```python
from build123d import *

# Parameters (mm, degrees)
F0_W      = 70
F0_H      = 100
F1_DEPTH  = 45
F2_W      = 60
F2_H      = 90
F3_DEPTH  = 40
F4_R      = 2.65
F5_DEPTH  = 5
F6_DEPTH  = 25
F7_DEPTH  = 25
F8_DEPTH  = 25
F9_W      = 5
F9_H      = 100
F10_DEPTH = 25
F11_W     = 5
F11_H     = 100
F12_DEPTH = 25
F14_DEPTH = 25
F15_DEPTH = 25
F17_DEPTH = 25
F18_W     = 67
F18_H     = 97
F18_W_2   = 63
F18_H_2   = 93
F19_DEPTH = 2
F13_W     = 5
F13_H     = 30
F20_DEPTH = 25
F16_W     = 5
F16_H     = 30
F21_DEPTH = 25
F22_R     = 5
F23_DEPTH = 25
F25_DEPTH = 100


with BuildPart() as f1:
    # F0 (on Front) → F1 (new body)
    with BuildSketch(Plane.XZ):
        with Locations((12.707982, -8.253274)):
            Rectangle(F0_W, F0_H)
    extrude(amount=F1_DEPTH)

    # F2 (on face) → F3 (cut)
    with BuildSketch(Plane.XZ.offset(45)):
        with Locations((12.707982, -8.253274)):
            Rectangle(F2_W, F2_H)
    extrude(amount=-F3_DEPTH, mode=Mode.SUBTRACT)

    # F4 (on face) → F5 (cut)
    with BuildSketch(Plane.XZ.offset(5)):
        with Locations((-9.792018, 29.246726)):
            Circle(F4_R)
    extrude(amount=-F5_DEPTH, mode=Mode.SUBTRACT)

    # F4 (on face) → F6 (cut)
    with BuildSketch(Plane.XZ.offset(5)):
        with Locations((35.207982, 29.246726)):
            Circle(F4_R)
    extrude(amount=-F6_DEPTH, mode=Mode.SUBTRACT)

    # F4 (on face) → F7 (cut)
    with BuildSketch(Plane.XZ.offset(5)):
        with Locations((35.207982, -45.753274)):
            Circle(F4_R)
    extrude(amount=-F7_DEPTH, mode=Mode.SUBTRACT)

    # F4 (on face) → F8 (cut)
    with BuildSketch(Plane.XZ.offset(5)):
        with Locations((-9.792018, -45.753274)):
            Circle(F4_R)
    extrude(amount=-F8_DEPTH, mode=Mode.SUBTRACT)

    # F9 (on face) → F10 (join)
    with BuildSketch(Plane(origin=(-22.292018, 0, 0), x_dir=(0, -1, 0), z_dir=(-1, 0, 0))):
        with Locations((2.5, -8.253274)):
            Rectangle(F9_W, F9_H)
    extrude(amount=F10_DEPTH)

    # F11 (on face) → F12 (join)
    with BuildSketch(Plane.YZ.offset(47.707982)):
        with Locations((-2.5, -8.253274)):
            Rectangle(F11_W, F11_H)
    extrude(amount=F12_DEPTH)

    # F13 (on face) → F14 (cut)
    with BuildSketch(Plane.XZ.offset(5)):
        with BuildLine():
            ThreePointArc((-47.292018, 16.746726), (-39.969687, 34.424395), (-22.292018, 41.746726))
            Line((-22.292018, 41.746726), (-47.292018, 41.746726))
            Line((-47.292018, 41.746726), (-47.292018, 16.746726))
        make_face()
    extrude(amount=-F14_DEPTH, mode=Mode.SUBTRACT)

    # F13 (on face) → F15 (cut)
    with BuildSketch(Plane.XZ.offset(5)):
        with BuildLine():
            Line((-47.292018, -58.253274), (-22.292018, -58.253274))
            ThreePointArc((-22.292018, -58.253274), (-39.969687, -50.930944), (-47.292018, -33.253274))
            Line((-47.292018, -33.253274), (-47.292018, -58.253274))
        make_face()
    extrude(amount=-F15_DEPTH, mode=Mode.SUBTRACT)

    # F16 (on face) → F17 (cut)
    with BuildSketch(Plane.XZ.offset(5)):
        with BuildLine():
            Line((72.707982, 41.746726), (47.707982, 41.746726))
            ThreePointArc((47.707982, 41.746726), (65.385652, 34.424395), (72.707982, 16.746726))
            Line((72.707982, 16.746726), (72.707982, 41.746726))
        make_face()
        with BuildLine():
            ThreePointArc((72.707982, -33.253274), (65.385652, -50.930944), (47.707982, -58.253274))
            Line((47.707982, -58.253274), (72.707982, -58.253274))
            Line((72.707982, -58.253274), (72.707982, -33.253274))
        make_face()
    extrude(amount=-F17_DEPTH, mode=Mode.SUBTRACT)

    # F18 (on face) → F19 (cut)
    with BuildSketch(Plane.XZ.offset(45)):
        with Locations((12.707982, -8.253274)):
            Rectangle(F18_W, F18_H)
        with Locations((12.707982, -8.253274)):
            Rectangle(F18_W_2, F18_H_2, mode=Mode.SUBTRACT)
    extrude(amount=-F19_DEPTH, mode=Mode.SUBTRACT)

    # F13 (on face) → F20 (cut)
    with BuildSketch(Plane.XZ.offset(5)):
        Polygon((-37.292018, 6.746726), (-42.292018, 6.746726), (-42.292018, -23.253274), (-37.288308, -23.253274), align=None)
        with Locations((-29.792018, -8.253274)):
            Rectangle(F13_W, F13_H)
    extrude(amount=-F20_DEPTH, mode=Mode.SUBTRACT)

    # F16 (on face) → F21 (cut)
    with BuildSketch(Plane.XZ.offset(5)):
        with Locations((55.207982, -8.253274)):
            Rectangle(F16_W, F16_H)
        with Locations((65.207982, -8.253274)):
            Rectangle(F16_W, F16_H)
    extrude(amount=-F21_DEPTH, mode=Mode.SUBTRACT)

    # F22 (on face) → F23 (cut)
    with BuildSketch(Plane(origin=(0, 0, -58.253274), x_dir=(1, 0, 0), z_dir=(0, 0, -1))):
        with Locations((30.207982, 22.5)):
            Circle(F22_R)
        with Locations((-4.792018, 22.5)):
            Circle(F22_R)
    extrude(amount=-F23_DEPTH, mode=Mode.SUBTRACT)

    # F24 (on face) → F25 (cut)
    with BuildSketch(Plane.XY.offset(41.746726)):
        with BuildLine():
            Line((22.267865, 0), (-2.053064, 0))
            ThreePointArc((-2.053064, 0), (10.1074, -2.837065), (22.267865, 0))
        make_face()
    extrude(amount=-F25_DEPTH, mode=Mode.SUBTRACT)


solid = f1.part
```
Geometry check sheet. Reference: the model listing, model coordinates, mm. A direction names the side the tool comes from. Round coordinates to 2 decimals unless told otherwise and drop trailing zeros. Order: outer loops, then holes, each group sorted by start corner. A loop starts at its lowest first (then second) coordinate and runs counter-clockwise, first axis right, second up. Notation, with made-up numbers: (26.5, 64) - (82.5, 64) arc R36 ccw to (82.5, 101) - close; hole circle Ø7 at (10, 24). An arc over 180 degrees is marked (long way). Use a Markdown table: item, result. Add a question column.
(1) Sectioned sample at C-C, the plane z = -25. Enter the section's corners in (x, y), and give its area (3 significant figures).
(2) Sectioned sample at D-D, the plane x = 3. Enter the section's corners in (y, z).
(3) Sectioned sample at B-B, the plane y = -22.5. Enter the section's corners in (x, z), and give its area (3 significant figures).
(4) Release check for a two-part mould opening along Z. For faces 5 (the cylindrical face through (-39.8, -2.5, -51.1)), 6 (the flat face through (-21, -45, -8)), 7 (the flat face through (-32.292, -3, -8)) record: pulls with the +Z half, pulls with the -Z half, needs draft (parallel to the pull), parting line crosses it, or undercut.
(5) Material ranges on line 1 along X through (y, z) = (-26.5, -7); line 2 along Z through (x, y) = (6, -32.5); line 3 along Y through (x, z) = (-15.5, -24), recorded low to high. Write a range as [from, to].
(6) Depth check by flat-ended pin: pin 1 (12.5 mm diameter, centred on x = 62.5, z = 7, fed in from -Y); pin 2 (1 mm diameter, centred on y = -43.5, z = 5, fed in from -X); pin 3 (1.5 mm diameter, centred on x = -39.5, y = -3.5, fed in from +Z). Enter the tip coordinate at first touch or a pass-through.
(7) Tool access check on faces 1 (the flat face through (52.708, -3, -8)), 2 (the flat face through (-35, -5, -9)), 3 (the cylindrical face through (29.12, -17.62, -55.79)), 4 (the flat face through (47.708, -25, -9)). Record the directions out of +Z, -Z, +X, -X, +Y, -Y that give a thin tool (end or side, any length) a straight path to the whole face; none if there is none.
(8) Sectioned sample at A-A, the plane y = -38.5. Enter the section's corners in (x, z).
Answers below:
| question | item | result |
|---|---|---|
| 1 | outline | (-47.29, -5) - (-22.29, -5) - (-22.29, -45) - (-20.79, -45) - (-20.79, -43) - (-18.79, -43) - (-18.79, -45) - (-17.29, -45) - (-17.29, -5) - (42.71, -5) - (42.71, -45) - (44.21, -45) - (44.21, -43) - (46.21, -43) - (46.21, -45) - (47.71, -45) - (47.71, -5) - (72.71, -5) - (72.71, 0) - (22.27, 0) arc R27.48 cw to (-2.05, 0) - (-47.29, 0) - close |
| 1 | area | 946 mm² |
| 2 | outline | (-45, -58.25) - (-1.9, -58.25) - (-1.9, 41.75) - (-45, 41.75) - (-45, 40.25) - (-43, 40.25) - (-43, 38.25) - (-45, 38.25) - (-45, 36.75) - (-5, 36.75) - (-5, -53.25) - (-45, -53.25) - (-45, -54.75) - (-43, -54.75) - (-43, -56.75) - (-45, -56.75) - close |
| 3 | outline | (-22.29, -58.25) - (-9.79, -58.25) - (-9.79, -53.25) - (-17.29, -53.25) - (-17.29, 36.75) - (42.71, 36.75) - (42.71, -53.25) - (35.21, -53.25) - (35.21, -58.25) - (47.71, -58.25) - (47.71, 41.75) - (-22.29, 41.75) - close; (0.21, -58.25) - (25.21, -58.25) - (25.21, -53.25) - (0.21, -53.25) - close |
| 3 | area | 1,500 mm² |
| 4 | face 5 | pulls with the -Z half |
| 4 | face 6 | needs draft |
| 4 | face 7 | undercut |
| 5 | line 1 | [-22.29, -17.29], [42.71, 47.71] |
| 5 | line 2 | [-58.25, -53.25], [36.75, 41.75] |
| 5 | line 3 | [-5, 0] |
| 6 | pin 1 | y = -5 |
| 6 | pin 2 | x = -22.29 |
| 6 | pin 3 | z = 35.57 |
| 7 | face 1 | +Y, -Y |
| 7 | face 2 | +Z, -Z, -X, -Y |
| 7 | face 3 | -Z |
| 7 | face 4 | +Z, -Z, +X, -Y |
| 8 | outline | (-22.29, -58.25) - (47.71, -58.25) - (47.71, 41.75) - (-22.29, 41.75) - close; hole (-17.29, -53.25) - (42.71, -53.25) - (42.71, 36.75) - (-17.29, 36.75) - close |
